Could you check a few things on this model? Use its own coordinates, in mm. Face numbers are marked on the shaded views. A direction names the side the tool comes from. Coordinates: 2 decimals unless noted, no trailing zeros. Loops run counter-clockwise (first coordinate to the right, second up) from the corner with the lowest first, then second, coordinate; pieces in that order, holes last. Notation, with made-up numbers: M 56,51.25 L 113,51.25 A23 ccw 113,74.25 Z; hole C -1,3.5 d6. An arc over 180 degrees is marked long. Use one line per item in the form item = value. Start each with the question number.
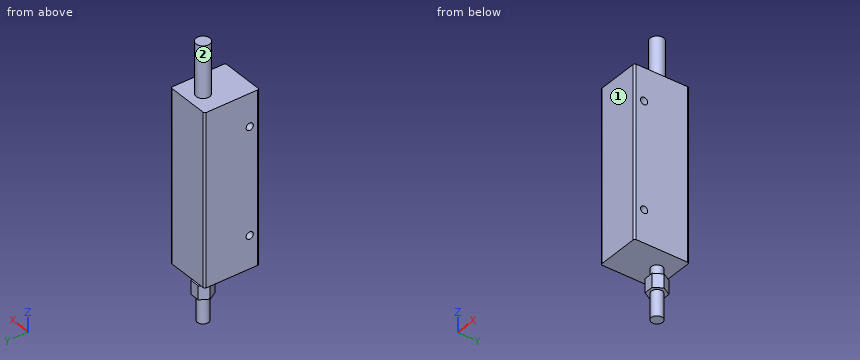
```python
from build123d import *

# Parameters (mm, degrees)
SKETCH1_W           = 13
SKETCH1_H           = 16
BOSS_EXTRUDE1_DEPTH = 50
SKETCH2_R           = 1.05
CUT_EXTRUDE1_DEPTH  = 55.083269132
SKETCH3_R           = 2
BOSS_EXTRUDE2_DEPTH = 15
SKETCH4_R           = 1.65
BOSS_EXTRUDE3_DEPTH = 14.5
FILLET1_R           = 0.5
BOSS_EXTRUDE4_START = -7.5
BOSS_EXTRUDE4_DEPTH = 4


with BuildPart() as part:
    # Sketch1 → Boss-Extrude1 (new body)
    with BuildSketch(Plane.XY):
        with Locations((6.5, 8)):
            Rectangle(SKETCH1_W, SKETCH1_H)
    extrude(amount=BOSS_EXTRUDE1_DEPTH)

    # Sketch2 → Cut-Extrude1 (cut, through all)
    with BuildSketch(Plane(origin=(13, 0, 0), x_dir=(0, 0, -1), z_dir=(1, 0, 0))):
        with Locations(Location((-40.5, 2.8, 0), (0, 0, 90))):
            Circle(SKETCH2_R)
        with Locations(Location((-9.5, 2.8, 0), (0, 0, 90))):
            Circle(SKETCH2_R)
    extrude(amount=-CUT_EXTRUDE1_DEPTH, mode=Mode.SUBTRACT)

    # Sketch3 → Boss-Extrude2 (add)
    with BuildSketch(Plane.XY.offset(50)):
        with Locations(Location((6.5, 11.5, 0), (0, 0, 180))):
            Circle(SKETCH3_R)
    extrude(amount=BOSS_EXTRUDE2_DEPTH)

    # Sketch4 → Boss-Extrude3 (add)
    with BuildSketch(Plane(origin=(0, 0, 0), x_dir=(-1, 0, 0), z_dir=(0, 0, -1))):
        with Locations(Location((-6.5, 11.5, 0), (0, 0, 180))):
            Circle(SKETCH4_R)
    extrude(amount=BOSS_EXTRUDE3_DEPTH)

    # Fillet1
    fillet1_edges = [part.edges().sort_by_distance(p)[0] for p in [
        (0, 16, 25),
        (13, 16, 25),
        (13, 0, 25),
        (0, 0, 25),
    ]]
    fillet(fillet1_edges, radius=FILLET1_R)

    # Sketch6 → Boss-Extrude4 (add)
    with BuildSketch(Plane(origin=(0, 0, -14.5), x_dir=(-1, 0, 0), z_dir=(0, 0, -1)).offset(BOSS_EXTRUDE4_START)):
        Polygon((-7.86221417, 9.070311134), (-5.076934804, 9.10544349), (-3.714720633, 11.535132356), (-5.13778583, 13.929688866), (-7.923065196, 13.89455651), (-9.285279367, 11.464867644), align=None)
    extrude(amount=-BOSS_EXTRUDE4_DEPTH)


solid = part.part
```
Item 1: For the marked faces 1 and 2, which set-ups out of +Z, -Z, +X, -X, +Y, -Y let a thin tool reach every point of the face, with its end or its side?
Item 2: I want a section at C-C (x = 3). Write out the boundary of the cut face in (y, z), plus the area to 3 significant figures.
Item 3: I want a section at B-B (y = 2.8). Write out the boundary of the cut face in (x, z), plus the area to 3 significant figures.
Item 4: I want a section at D-D (z = 59.5). Write out the boundary of the cut face in (x, y).
Item 5: I want a section at A-A (z = 40.5). Write out the boundary of the cut face in (x, y), plus the area to 3 significant figures.
Item 6: I'm going to push flat-ended pins straight in: P1, Ø1.5, axis at x = 11.5, y = 3.5, coming from the +Z side; P2, Ø4, axis at x = 4, y = 7.5, coming from the -Z side. Where does each tip first touch, or does it pass through?
Item 7: Please list where these lines run through material, in increasing order: line 1 along Z through (x, y) = (8, 2.8); line 2 along Z through (x, y) = (0.5, 8); line 3 along X through (y, z) = (13.25, 55).
Worked answers:
q1.face_1 = +Z, -Z, +X, -X, -Y
q1.face_2 = +Z
q2.outline = M 0,0 L 16,0 L 16,50 L 0,50 Z; hole C 2.8,9.5 d2.1; hole C 2.8,40.5 d2.1
q2.area = 793 mm²
q3.outline = M 0,0 L 13,0 L 13,8.45 L 0,8.45 Z; M 0,10.55 L 13,10.55 L 13,39.45 L 0,39.45 Z; M 0,41.55 L 13,41.55 L 13,50 L 0,50 Z
q3.area = 595 mm²
q4.outline = C 6.5,11.5 d4
q5.outline = M 0,0.5 A0.5 ccw 0.5,0 L 12.5,0 A0.5 ccw 13,0.5 L 13,1.75 L 0,1.75 Z; M 0,3.85 L 13,3.85 L 13,15.5 A0.5 ccw 12.5,16 L 0.5,16 A0.5 ccw 0,15.5 Z
q5.area = 180 mm²
q6.P1 = 50
q6.P2 = -7
q7.line_1 = 0 to 8.45, 10.55 to 39.45, 41.55 to 50
q7.line_2 = 0 to 50
q7.line_3 = 5.53 to 7.47
